Check sheet for the modelled part. Datum: model origin and axes. Units: mm. A direction names the side the tool comes from. Coordinates: 2 decimals unless noted, no trailing zeros. Loops run counter-clockwise (first coordinate to the right, second up) from the corner with the lowest first, then second, coordinate; pieces in that order, holes last.
```python
from build123d import *

# Parameters (mm, degrees)
SKETCH_1_W             = 17.9
SKETCH_1_H             = 8
EXTRUDE_1_DEPTH        = 100
SKETCH_2_R             = 1.5
CUT_EXTRUDE_1_DEPTH    = 100
HOLE_WIZARD_M5_1_D     = 4.2
HOLE_WIZARD_M5_1_DEPTH = 12.4
HOLE_WIZARD_M5_1_TIP   = 1.2618073
CHAMFER_1_SIZE         = 1
FILLET_1_R             = 2
HOLE_WIZARD_M5_2_D     = 4.2
HOLE_WIZARD_M5_2_DEPTH = 12.4
HOLE_WIZARD_M5_2_TIP   = 1.2618073
CUT_EXTRUDE_2_DEPTH    = 10


with BuildPart() as part:
    # 草图1 → 凸台-拉伸1 (new, symmetric)
    with BuildSketch(Plane.XY):
        Rectangle(SKETCH_1_W, SKETCH_1_H)
    extrude(amount=EXTRUDE_1_DEPTH, both=True)

    # 草图2 → 切除-拉伸1 (cut, symmetric)
    with BuildSketch(Plane(origin=(0, 4, 0), x_dir=(1, 0, 0), z_dir=(0, 1, 0))):
        with Locations(Location((0, 90, 0), (0, 0, 270))):
            Circle(SKETCH_2_R)
        with Locations(Location((0, 45, 0), (0, 0, 270))):
            Circle(SKETCH_2_R)
        with Locations(Location((0, 0, 0), (0, 0, 270))):
            Circle(SKETCH_2_R)
        with Locations(Location((0, -45, 0), (0, 0, 270))):
            Circle(SKETCH_2_R)
        with Locations(Location((0, -90, 0), (0, 0, 270))):
            Circle(SKETCH_2_R)
    extrude(amount=CUT_EXTRUDE_1_DEPTH, both=True, mode=Mode.SUBTRACT)

    # M5 螺纹孔1
    with Locations(Plane(origin=(0, 4, 0), x_dir=(1, 0, 0), z_dir=(0, 1, 0))):
        with Locations((0, 90), (0, 45), (0, 0), (0, -45), (0, -90)):
            Hole(HOLE_WIZARD_M5_1_D / 2, depth=HOLE_WIZARD_M5_1_DEPTH)
            with Locations((0, 0, -(HOLE_WIZARD_M5_1_DEPTH + HOLE_WIZARD_M5_1_TIP / 2))):  # 118° drill point
                Cone(0, HOLE_WIZARD_M5_1_D / 2, HOLE_WIZARD_M5_1_TIP, mode=Mode.SUBTRACT)

    # 倒角1
    chamfer_1_edges = [part.edges().sort_by_distance(p)[0] for p in [
        (8.95, -4, 0),
        (-8.95, -4, 0),
        (-8.95, 4, 0),
        (8.95, 4, 0),
    ]]
    chamfer(chamfer_1_edges, length=CHAMFER_1_SIZE)

    # 圆角1
    fillet_1_edges = [part.edges().sort_by_distance(p)[0] for p in [
        (8.95, 0, -100),
        (-8.95, 0, -100),
        (-8.95, 0, 100),
        (8.95, 0, 100),
    ]]
    fillet(fillet_1_edges, radius=FILLET_1_R)

    # M5 螺纹孔2
    with Locations(Plane(origin=(0, 4, 0), x_dir=(1, 0, 0), z_dir=(0, 1, 0))):
        with Locations((0, 67.5), (0, 22.5), (0, -22.5), (0, -67.5)):
            Hole(HOLE_WIZARD_M5_2_D / 2, depth=HOLE_WIZARD_M5_2_DEPTH)
            with Locations((0, 0, -(HOLE_WIZARD_M5_2_DEPTH + HOLE_WIZARD_M5_2_TIP / 2))):  # 118° drill point
                Cone(0, HOLE_WIZARD_M5_2_D / 2, HOLE_WIZARD_M5_2_TIP, mode=Mode.SUBTRACT)

    # 草图8 → 切除-拉伸2 (cut)
    with BuildSketch(Plane(origin=(0, 4, 0), x_dir=(1, 0, 0), z_dir=(0, 1, 0))):
        with BuildLine():
            Line((3, 82.75), (3, 74.75))
            ThreePointArc((3, 74.75), (0, 71.75), (-3, 74.75))
            Line((-3, 74.75), (-3, 82.75))
            ThreePointArc((-3, 82.75), (0, 85.75), (3, 82.75))
        make_face()
        with BuildLine():
            Line((3, 60.4), (3, 52.4))
            ThreePointArc((3, 52.4), (0, 49.4), (-3, 52.4))
            Line((-3, 52.4), (-3, 60.4))
            ThreePointArc((-3, 60.4), (0, 63.4), (3, 60.4))
        make_face()
        with BuildLine():
            Line((3, 38.05), (3, 30.05))
            ThreePointArc((3, 30.05), (0, 27.05), (-3, 30.05))
            Line((-3, 30.05), (-3, 38.05))
            ThreePointArc((-3, 38.05), (0, 41.05), (3, 38.05))
        make_face()
        with BuildLine():
            Line((3, 15.7), (3, 7.7))
            ThreePointArc((3, 7.7), (0, 4.7), (-3, 7.7))
            Line((-3, 7.7), (-3, 15.7))
            ThreePointArc((-3, 15.7), (0, 18.7), (3, 15.7))
        make_face()
        with BuildLine():
            Line((3, -6.65), (3, -14.65))
            ThreePointArc((3, -14.65), (0, -17.65), (-3, -14.65))
            Line((-3, -14.65), (-3, -6.65))
            ThreePointArc((-3, -6.65), (0, -3.65), (3, -6.65))
        make_face()
        with BuildLine():
            Line((3, -29), (3, -37))
            ThreePointArc((3, -37), (0, -40), (-3, -37))
            Line((-3, -37), (-3, -29))
            ThreePointArc((-3, -29), (0, -26), (3, -29))
        make_face()
        with BuildLine():
            Line((3, -51.35), (3, -59.35))
            ThreePointArc((3, -59.35), (0, -62.35), (-3, -59.35))
            Line((-3, -59.35), (-3, -51.35))
            ThreePointArc((-3, -51.35), (0, -48.35), (3, -51.35))
        make_face()
        with BuildLine():
            Line((3, -73.7), (3, -81.7))
            ThreePointArc((3, -81.7), (0, -84.7), (-3, -81.7))
            Line((-3, -81.7), (-3, -73.7))
            ThreePointArc((-3, -73.7), (0, -70.7), (3, -73.7))
        make_face()
    extrude(amount=-CUT_EXTRUDE_2_DEPTH, mode=Mode.SUBTRACT)


solid = part.part
```
1) Depth check by flat-ended pin: pin 1 (8 mm diameter, centred on x = 2, z = -60.5, fed in from +Y). Enter the tip coordinate at first touch or a pass-through.
Answer sheet:
pin 1: stops at y = 4
2) Scan lines: line 1 (X direction, y = 2, z = 56); line 2 (X direction, y = 2.25, z = 45). Record each from-to range of solid material in increasing order.
Answer sheet:
line 1: x = -8.95 to -3, 3 to 8.95
line 2: x = -8.95 to -2.1, 2.1 to 8.95
3) Section check A-A on z = 0. Enter the section's corners in (x, y), plus the area to 3 significant figures.
Answer sheet:
outline: (-8.95, -3) - (-7.95, -4) - (-2.1, -4) - (-2.1, 4) - (-7.95, 4) - (-8.95, 3) - close; (2.1, -4) - (7.95, -4) - (8.95, -3) - (8.95, 3) - (7.95, 4) - (2.1, 4) - close
area: 108 mm2
4) Set-up check for faces 1 (the flat face through (3, 0, 55)), 2 (the flat face through (0, 0, -100)): record each of +Z, -Z, +X, -X, +Y, -Y from which the full face is reachable in a straight line by a thin tool's end or side.
Answer sheet:
face 1: +Y, -Y
face 2: -Z, +X, -X, +Y, -Y
5) Section check B-B on x = 0. Give the number of separate pieces and of enclosed holes in the cut face, plus the area to 3 significant figures.
Answer sheet:
separate pieces: 18
enclosed holes: 0
area: 402 mm2
